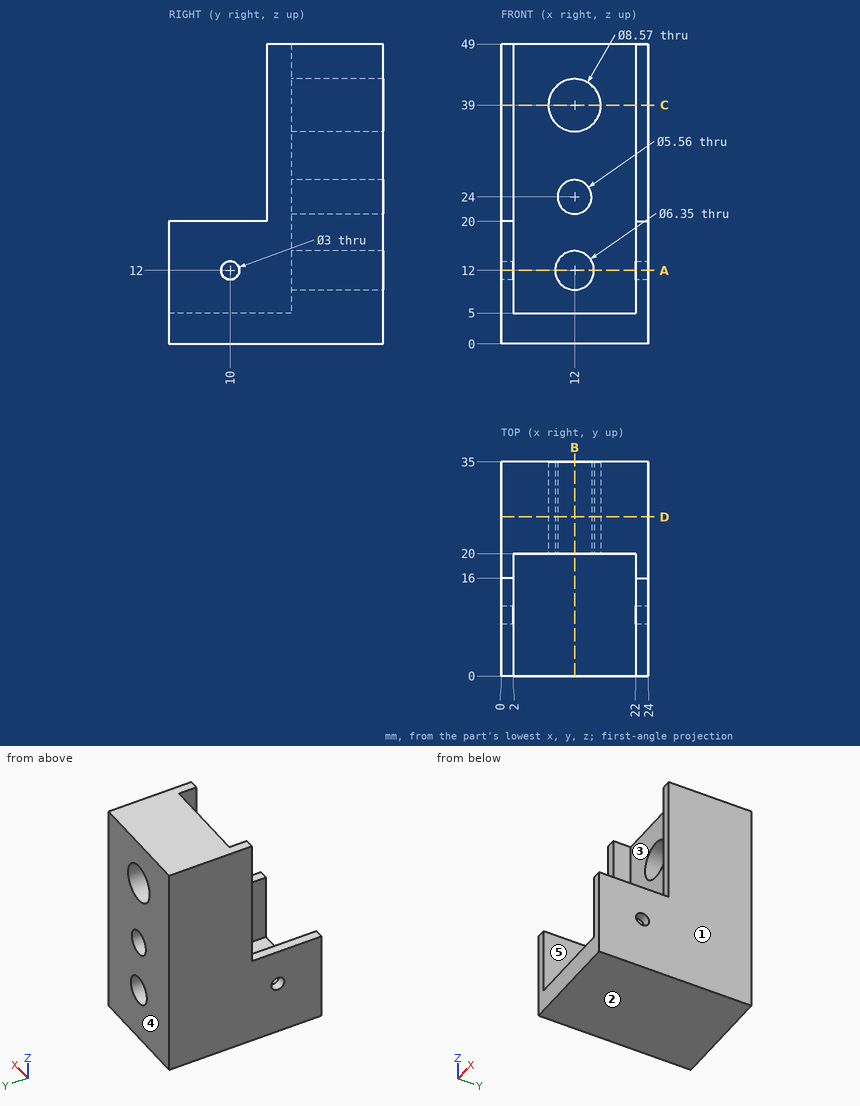
Part print with two shaded views. Sizes in mm from the minimum x, y, z corner. A direction names the side the tool comes from. Round coordinates to 2 decimals unless told otherwise and drop trailing zeros. Order: outer loops, then holes, each group sorted by start corner. A loop starts at its lowest first (then second) coordinate and runs counter-clockwise, first axis right, second up.
(1) Band-saw the part on D-D (y = 26). List the corners of the cut face in (x, z) (3 decimals).
(2) Drill centre lines: line 1 (X direction, y = 4, z = 13); line 2 (X direction, y = 30, z = 12) (3 decimals); line 3 (Z direction, x = 15, y = 9). Where is each one in solid material? Low to high.
(3) Band-saw the part on C-C (z = 39). List the corners of the cut face in (x, y) (3 decimals).
(4) Band-saw the part on A-A (z = 12). List the corners of the cut face in (x, y) (3 decimals), then the cut area to 3 significant figures.
(5) Pin check, flat tips, straight feed: pin 1 (0.6 mm diameter, centred on x = 23.5, z = 33, fed in from -Y); pin 2 (5 mm diameter, centred on x = 7.5, y = 4.5, fed in from +Z); pin 3 (1.6 mm diameter, centred on x = 23.5, y = 6.5, fed in from +Z). Stop position of each tip, or through.
(6) Pull direction X, two halves, no side cores. Call the marked faces 1, 2 and 3: released by +X, released by -X, zero draft, split by the parting line, or undercut.
(7) 3-axis set-ups, long thin cutter, end or side, ignore diameter. For the marked faces 4 and 5: which of +Z, -Z, +X, -X, +Y, -Y reach the whole face in a straight line?
(8) Band-saw the part on B-B (x = 12). List the corners of the cut face in (y, z) (3 decimals).
Verdict:
1. outline: (0, 0) - (24, 0) - (24, 49) - (0, 49) - close; hole circle Ø8.57 at (12, 39); hole circle Ø6.35 at (12, 12); hole circle Ø5.56 at (12, 24)
2. line 1: x = 0 to 2, 22 to 24
2. line 2: x = 0 to 8.825, 15.175 to 24
2. line 3: z = 0 to 5
3. outline: (0, 16) - (2, 16) - (2, 20) - (7.715, 20) - (7.715, 35) - (0, 35) - close; (16.285, 20) - (22, 20) - (22, 16) - (24, 16) - (24, 35) - (16.285, 35) - close
4. outline: (0, 0) - (2, 0) - (2, 8.5) - (0, 8.5) - close; (0, 11.5) - (2, 11.5) - (2, 20) - (8.825, 20) - (8.825, 35) - (0, 35) - close; (15.175, 20) - (22, 20) - (22, 11.5) - (24, 11.5) - (24, 35) - (15.175, 35) - close; (22, 0) - (24, 0) - (24, 8.5) - (22, 8.5) - close
4. area: 333 mm2
5. pin 1: stops at y = 16
5. pin 2: stops at z = 5
5. pin 3: stops at z = 20
6. face 1: released by +X
6. face 2: zero draft
6. face 3: undercut
7. face 4: +Z, -Z, +X, -X, +Y
7. face 5: +Z, -Y
8. outline: (0, 0) - (35, 0) - (35, 8.825) - (20, 8.825) - (20, 5) - (0, 5) - close; (20, 15.175) - (35, 15.175) - (35, 21.22) - (20, 21.22) - close; (20, 26.78) - (35, 26.78) - (35, 34.715) - (20, 34.715) - close; (20, 43.285) - (35, 43.285) - (35, 49) - (20, 49) - close
